from build123d import *

# Parameters (mm, degrees)
ESQUISSE1_W        = 25
ESQUISSE1_H        = 55
BOSS_EXTRU_1_DEPTH = 2
ESQUISSE2_W        = 25
ESQUISSE2_H        = 2
BOSS_EXTRU_2_DEPTH = 53
BOSS_EXTRU_3_DEPTH = 2
ESQUISSE6_W        = 38
ESQUISSE6_H        = 60
BOSS_EXTRU_4_DEPTH = 2
ESQUISSE7_W        = 40
ESQUISSE7_H        = 40
BOSS_EXTRU_5_DEPTH = 20
ESQUISSE9_W        = 2
ESQUISSE9_H        = 40
BOSS_EXTRU_6_DEPTH = 25
ESQUISSE8_R        = 4.5
BOSS_EXTRU_7_DEPTH = 7


with BuildPart() as part:
    # Esquisse1 → Boss.-Extru.1 (new body)
    with BuildSketch(Plane(origin=(0, 0, 0), x_dir=(1, 0, 0), z_dir=(0, 1, 0))):
        with Locations((12.5, 27.5)):
            Rectangle(ESQUISSE1_W, ESQUISSE1_H)
    extrude(amount=BOSS_EXTRU_1_DEPTH)

    # Esquisse2 → Boss.-Extru.2 (add)
    with BuildSketch(Plane(origin=(0, 2, 0), x_dir=(1, 0, 0), z_dir=(0, 1, 0))):
        with Locations((12.5, 54)):
            Rectangle(ESQUISSE2_W, ESQUISSE2_H)
    extrude(amount=BOSS_EXTRU_2_DEPTH)

    # Esquisse3 → Boss.-Extru.3 (add)
    with BuildSketch(Plane.XY.offset(-53)):
        with BuildLine():
            Line((0, 2), (25, 2))
            Line((25, 2), (25, 55))
            ThreePointArc((25, 55), (12.5, 67.5), (0, 55))
            Line((0, 55), (0, 2))
        make_face()
    extrude(amount=-BOSS_EXTRU_3_DEPTH)

    # Esquisse6 → Boss.-Extru.4 (add)
    with BuildSketch(Plane(origin=(0, 0, -55), x_dir=(-1, 0, 0), z_dir=(0, 0, -1))):
        with Locations((-16, 55.5)):
            Rectangle(ESQUISSE6_W, ESQUISSE6_H)
    extrude(amount=BOSS_EXTRU_4_DEPTH)

    # Esquisse7 → Boss.-Extru.5 (add)
    with BuildSketch(Plane(origin=(0, 0, -57), x_dir=(-1, 0, 0), z_dir=(0, 0, -1))):
        with Locations((-23, 55.5)):
            Rectangle(ESQUISSE7_W, ESQUISSE7_H)
    extrude(amount=BOSS_EXTRU_5_DEPTH)

    # Esquisse9 → Boss.-Extru.6 (add)
    with BuildSketch(Plane(origin=(0, 0, -57), x_dir=(-1, 0, 0), z_dir=(0, 0, -1))):
        with Locations((2, 59.5)):
            Rectangle(ESQUISSE9_W, ESQUISSE9_H)
    extrude(amount=BOSS_EXTRU_6_DEPTH)

    # Esquisse8 → Boss.-Extru.7 (add)
    with BuildSketch(Plane(origin=(43, 0, 0), x_dir=(0, 0, -1), z_dir=(1, 0, 0))):
        with Locations(Location((67, 66, 0), (0, 0, 180))):
            Circle(ESQUISSE8_R)
    extrude(amount=BOSS_EXTRU_7_DEPTH)


solid = part.part
Build history of the part. All positions in model axes, mm. A direction names the side the tool comes from. Coordinates: 2 decimals unless noted, no trailing zeros. Order: outer loops, then holes, each group sorted by start corner. A loop starts at its lowest first (then second) coordinate and runs counter-clockwise, first axis right, second up. Notation, with made-up numbers: (-6, 64.5) - (20, 64.5) arc R24 ccw to (20, 75.5) - close; hole circle Ø8 at (15.5, 80.5). An arc over 180 degrees is marked (long way). Put each result on its own line as item: value.
1. Saw through at C-C (y = 34). Write the cut outline in (x, z), and give its area (3 significant figures).
Answer sheet:
outline: (-3, -57) - (35, -57) - (35, -55) - (25, -55) - (25, -53) - (0, -53) - (0, -55) - (-3, -55) - close
area: 126 mm^2
2. Saw through at D-D (x = 20). Write the cut outline in (y, z), and give its area (3 significant figures).
Answer sheet:
outline: (0, -55) - (25.5, -55) - (25.5, -57) - (35.5, -57) - (35.5, -77) - (75.5, -77) - (75.5, -57) - (85.5, -57) - (85.5, -55) - (65, -55) - (65, -53) - (2, -53) - (2, 0) - (0, 0) - close
area: 1,160 mm^2
3. Tool access for faces 1 (the face through (0, 15, -54)), 2 (the face through (46.451, 62.206, -64.581)), 3 (the face through (39, 56, -57)): list every direction of +Z, -Z, +X, -X, +Y, -Y with a clear straight run to the whole face (end or side of a thin tool).
Answer sheet:
face 1: +Z, -X, +Y, -Y
face 2: +X
face 3: +Z, +X, +Y, -Y
4. Saw through at B-B (z = -67). Write the cut outline in (x, y), and give its area (3 significant figures).
Answer sheet:
outline: (-3, 39.5) - (-1, 39.5) - (-1, 79.5) - (-3, 79.5) - close; (3, 35.5) - (43, 35.5) - (43, 61.5) - (50, 61.5) - (50, 70.5) - (43, 70.5) - (43, 75.5) - (3, 75.5) - close
area: 1,740 mm^2
5. Saw through at A-A (x = 12.5). Write the cut outline in (y, z), and give its area (3 significant figures).
Answer sheet:
outline: (0, -55) - (25.5, -55) - (25.5, -57) - (35.5, -57) - (35.5, -77) - (75.5, -77) - (75.5, -57) - (85.5, -57) - (85.5, -55) - (67.5, -55) - (67.5, -53) - (2, -53) - (2, 0) - (0, 0) - close
area: 1,160 mm^2
6. Drop flat-ended pins along their axis: P1, Ø6, axis at x = 12, y = 65.5, coming from the +Z side; P2, Ø2, axis at y = 47.5, z = -58, coming from the +X side; P3, Ø2, axis at x = -2.5, z = -74.5, coming from the +Y side. Give the stop position or say it passes through.
Answer sheet:
P1: stops at z = -53
P2: stops at x = 43
P3: stops at y = 79.5
7. Probe line 1 along X through (y, z) = (52, -66); line 2 along Z through (x, y) = (17, 69); line 3 along Z through (x, y) = (16.5, 37). List the from-to ranges inside material, lowest first. Write a range as [from, to].
Answer sheet:
line 1: x = [-3, -1], [3, 43]
line 2: z = [-77, -55]
line 3: z = [-77, -53]
